For this review, use the dimensioned drawing (mm, ordinates from the lowest corner) and the shaded views. A direction names the side the tool comes from. Coordinates: 2 decimals unless noted, no trailing zeros. Return JSON: item names as keys, results as strings. Group by question number.
Item 1: Draft analysis for pull direction Z (two halves, no side actions). For the marked faces 1, 2 and 3, state which applies: +Z half, -Z half, draft (parallel to the pull), parting line (faces both ways), or undercut.
Item 2: Machinability: for the marked faces 4 and 5, which of the approach directions +Z, -Z, +X, -X, +Y, -Y give a long, thin tool a straight path to every point of the face, cutting with its end or side? Answer none if there is none.
Item 3: Insertion check: pin 1 (6 mm diameter, centred on x = 5.08, z = 5.08, fed in from +Y); pin 2 (2 mm diameter, centred on x = 5.5, z = 6, fed in from +Y); pin 3 (1.5 mm diameter, centred on x = 8, y = 2, fed in from +Z); pin 4 (1.5 mm diameter, centred on x = 1.5, z = 7, fed in from -Y). Each pin has a flat end and moves straight along its axis. Give the tip position at first contact, or say it passes through.
Item 4: For line 1 along Z through (x, y) = (5.08, 0.45) (1 decimal); line 2 along Y through (x, z) = (7.25, 7.5), list the stretches that pass through material, from the lowest coordinate up.
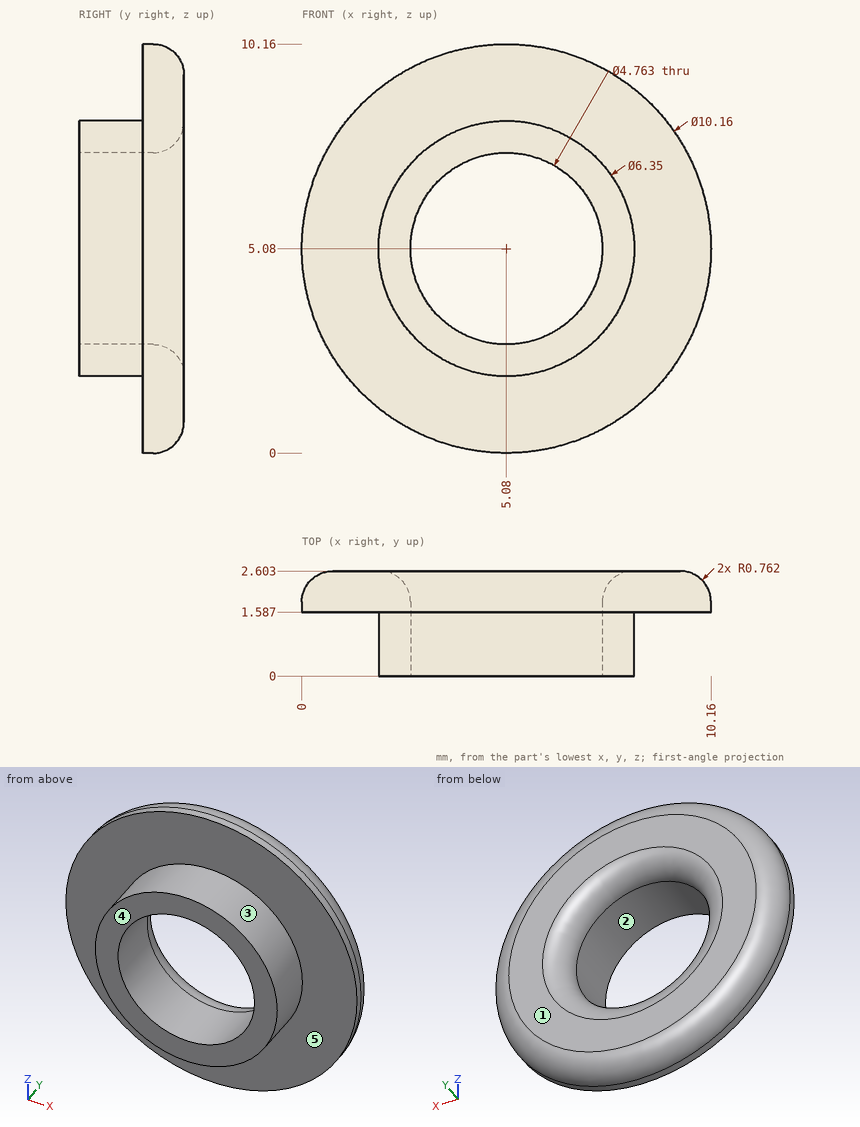
Findings below:
{
 "1": {"face 1": "draft", "face 2": "undercut", "face 3": "parting line"},
 "2": {"face 4": "+Z, -Z, +X, -X, -Y", "face 5": "-Y"},
 "3": {"pin 1": "stops at y = 2.59", "pin 2": "passes through", "pin 3": "stops at z = 9.67", "pin 4": "stops at y = 1.59"},
 "4": {"line 1": "z = 1.9 to 2.7, 7.5 to 8.3", "line 2": "y = 1.59 to 2.6"}
}
